from build123d import *

# Parameters (mm, degrees)
SKETCH1_W           = 30.2
SKETCH1_H           = 30.2
BOSS_EXTRUDE1_DEPTH = 1.6
SKETCH2_R           = 13.5
SKETCH2_R_2         = 12.5
BOSS_EXTRUDE2_DEPTH = 1
SKETCH3_R           = 1.1
CUT_EXTRUDE1_DEPTH  = 1


with BuildPart() as part:
    # Sketch1 → Boss-Extrude1 (new body)
    with BuildSketch(Plane(origin=(0, 0, 0), x_dir=(1, 0, 0), z_dir=(0, 1, 0))):
        with Locations((-27.198924567, -19.439049917)):
            Rectangle(SKETCH1_W, SKETCH1_H)
    extrude(amount=BOSS_EXTRUDE1_DEPTH)

    # Sketch2 → Boss-Extrude2 (add)
    with BuildSketch(Plane(origin=(0, 1.6, 0), x_dir=(1, 0, 0), z_dir=(0, 1, 0))):
        with Locations(Location((-27.198924567, -19.439049917, 0), (0, 0, 270))):
            Circle(SKETCH2_R)
        with Locations(Location((-27.198924567, -19.439049917, 0), (0, 0, 270))):
            Circle(SKETCH2_R_2, mode=Mode.SUBTRACT)
    extrude(amount=BOSS_EXTRUDE2_DEPTH)

    # Sketch3 → Cut-Extrude1 (cut)
    with BuildSketch(Plane(origin=(0, 1.6, 0), x_dir=(1, 0, 0), z_dir=(0, 1, 0))):
        with Locations(Location((-40.698924567, -32.939049917, 0), (0, 0, 270))):
            Circle(SKETCH3_R)
        with Locations(Location((-13.698924567, -32.939049917, 0), (0, 0, 270))):
            Circle(SKETCH3_R)
        with Locations(Location((-13.698924567, -5.939049917, 0), (0, 0, 270))):
            Circle(SKETCH3_R)
        with Locations(Location((-40.698924567, -5.939049917, 0), (0, 0, 270))):
            Circle(SKETCH3_R)
    extrude(amount=-CUT_EXTRUDE1_DEPTH, mode=Mode.SUBTRACT)


solid = part.part
Geometry: final body of the model. Coordinates: model frame, mm. A direction names the side the tool comes from. Coordinates: 2 decimals unless noted, no trailing zeros. Order: outer loops, then holes, each group sorted by start corner. A loop starts at its lowest first (then second) coordinate and runs counter-clockwise, first axis right, second up.
1) Draft query along Z for faces 3 (the flat face through (-27, 1, 4.339)), 4 (the cylindrical face through (-13.37, 1.11, 33.99)), 5 (the cylindrical face through (-13.37, 1.11, 6.99)), 6 (the flat face through (-12.099, 1, 20)). Return one class per face: released by +Z, released by -Z, zero draft, split by the parting line, or undercut.
Result sheet:
face 3: released by -Z
face 4: undercut
face 5: undercut
face 6: zero draft
2) Ray query, probe 1 along Z at (x, y) = (-13.5, 0.7); probe 2 along X at (y, z) = (0.95, 32); probe 3 along Y at (x, z) = (-16.5, 28.5). Return the intervals inside material, ascending.
Result sheet:
probe 1: z = 4.34 to 4.86, 7.02 to 31.86, 34.02 to 34.54
probe 2: x = -42.3 to -41.27, -40.13 to -14.27, -13.13 to -12.1
probe 3: y = 0 to 1.6
3) First-contact query: P1, Ø0.7, axis at x = -40, z = 33, coming from the +Y side; P2, Ø1.8, axis at x = -13.5, z = 6.5, coming from the +Y side. Flat tips, straight axial feed; report the tip coordinate or a pass-through.
Result sheet:
P1: stops at y = 0.6
P2: stops at y = 1.6
4) Section A-A (y = 1.05). Return loops of the section in (x, z).
Result sheet:
outline: (-42.3, 4.34) - (-12.1, 4.34) - (-12.1, 34.54) - (-42.3, 34.54) - close; hole circle Ø2.2 at (-40.7, 5.94); hole circle Ø2.2 at (-40.7, 32.94); hole circle Ø2.2 at (-13.7, 5.94); hole circle Ø2.2 at (-13.7, 32.94)
5) Section C-C (x = -19). Return loops of the section in (y, z).
Result sheet:
outline: (0, 4.34) - (1.6, 4.34) - (1.6, 8.71) - (2.6, 8.71) - (2.6, 10) - (1.6, 10) - (1.6, 28.87) - (2.6, 28.87) - (2.6, 30.16) - (1.6, 30.16) - (1.6, 34.54) - (0, 34.54) - close
6) Section B-B (z = 14.5). Return loops of the section in (x, y), then the cut area to 3 significant figures.
Result sheet:
outline: (-42.3, 0) - (-12.1, 0) - (-12.1, 1.6) - (-14.63, 1.6) - (-14.63, 2.6) - (-15.72, 2.6) - (-15.72, 1.6) - (-38.68, 1.6) - (-38.68, 2.6) - (-39.76, 2.6) - (-39.76, 1.6) - (-42.3, 1.6) - close
area: 50.5 mm2
7) Set-up query: faces 1 (the flat face through (-37.1, 2.6, 27.4)), 2 (the cylindrical face through (-14.805, 2.093, 17.812)). Return all of +Z, -Z, +X, -X, +Y, -Y with unobstructed straight access to the full face (end or side cutting, diameter ignored); none if empty.
Result sheet:
face 1: +Z, -Z, +X, -X, +Y
face 2: +Y
